Work out the finished part from the listing and answer in its coordinate system (mm). A direction names the side the tool comes from. Coordinates: 2 decimals unless noted, no trailing zeros. Write each loop counter-clockwise with the first axis right and the second up, starting at its lowest first coordinate (ties: lowest second). Pieces come first, ordered by that corner, then holes. Notation, with made-up numbers: (65.5, 55.25) - (101.5, 55.25) arc R18 cw to (101.5, 60.25) - close; hole circle Ø11 at (12, 80). An arc over 180 degrees is marked (long way). Use a Markdown table: item, result. Add a question column.
(1) The part is cut by section D-D, the plane x = -53. Give the vertices of the cut face in (y, z), then the cut area to 3 significant figures.
(2) Find the intervals of material crossed by line 1 (Y direction, x = 53, z = 1.1); line 2 (Z direction, x = -28, y = 0.5); line 3 (X direction, y = 3.25, z = -0.5), in increasing order. Write a range as from..to.
(3) For a pull along X with two mould halves and no side action, classify faces 3 (the face through (60, 0, 2)), 4 (the face through (4.846, -3.549, 1.972)), 5 (the face through (-1, 2, 4)) as released by +X, released by -X, zero draft, split by the parting line, or undercut.
(4) The part is cut by section B-B, the plane y = 0. Give the vertices of the cut face in (x, z), then the cut area to 3 significant figures.
(5) Given pin 1 Ø4 at (x, y) = (-11, -1.5) entering from -Z; pin 2 Ø6.5 at (x, y) = (53, 0) entering from +Z; pin 3 Ø8 at (y, z) = (-3.5, -8.5) entering from -X; pin 4 Ø1 at (y, z) = (-0.5, -2) entering from +X, each flat-ended and moving along its own axis, determine where each tip first touches the part or whether it passes through.
(6) The part is cut by section A-A, the plane x = 53. Give the vertices of the cut face in (y, z).
(7) The part is cut by section C-C, the plane z = 2. Give the vertices of the cut face in (x, y), then the cut area to 3 significant figures.
(8) A tool of negligible diameter and unlimited length cuts with its end or side. For faces 1 (the face through (-58, 0, -7)), 2 (the face through (-53, 0, -15)), from which of +Z, -Z, +X, -X, +Y, -Y can it reach the whole face along a straight path? Write none if from no direction.
from build123d import *

# Parameters (mm, degrees)
F0_W     = 120
F0_H     = 14
F0_R     = 5
F0_R_2   = 4
F1_DEPTH = 4
F2_DEPTH = 15


with BuildPart() as f1:
    # F0 (on Top) → F1 (new body)
    with BuildSketch(Plane.XY):
        Rectangle(F0_W, F0_H)
        with Locations((-53, 0)):
            Circle(F0_R, mode=Mode.SUBTRACT)
        with Locations((3, 0)):
            Circle(F0_R_2, mode=Mode.SUBTRACT)
        with Locations((53, 0)):
            Circle(F0_R_2, mode=Mode.SUBTRACT)
        with Locations((-53, 0)):
            Circle(F0_R)
    extrude(amount=F1_DEPTH)

    # F0 (on Top) → F2 (join)
    with BuildSketch(Plane.XY):
        with Locations((-53, 0)):
            Circle(F0_R)
    extrude(amount=-F2_DEPTH)


solid = f1.part
Model answer:
| question | item | result |
|---|---|---|
| 1 | outline | (-7, 0) - (-5, 0) - (-5, -15) - (5, -15) - (5, 0) - (7, 0) - (7, 4) - (-7, 4) - close |
| 1 | area | 206 mm^2 |
| 2 | line 1 | -7..-4, 4..7 |
| 2 | line 2 | 0..4 |
| 2 | line 3 | -56.8..-49.2 |
| 3 | face 3 | released by +X |
| 3 | face 4 | undercut |
| 3 | face 5 | zero draft |
| 4 | outline | (-60, 0) - (-58, 0) - (-58, -15) - (-48, -15) - (-48, 0) - (-1, 0) - (-1, 4) - (-60, 4) - close; (7, 0) - (49, 0) - (49, 4) - (7, 4) - close; (57, 0) - (60, 0) - (60, 4) - (57, 4) - close |
| 4 | area | 566 mm^2 |
| 5 | pin 1 | z = 0 |
| 5 | pin 2 | through |
| 5 | pin 3 | x = -58 |
| 5 | pin 4 | x = -48 |
| 6 | outline | (-7, 0) - (-4, 0) - (-4, 4) - (-7, 4) - close; (4, 0) - (7, 0) - (7, 4) - (4, 4) - close |
| 7 | outline | (-60, -7) - (60, -7) - (60, 7) - (-60, 7) - close; hole circle Ø8 at (3, 0); hole circle Ø8 at (53, 0) |
| 7 | area | 1,580 mm^2 |
| 8 | face 1 | -Z |
| 8 | face 2 | -Z, +X, -X, +Y, -Y |
